Build history of the part. All positions in model axes, mm. Round coordinates to 2 decimals unless told otherwise and drop trailing zeros. Write each loop counter-clockwise with the first axis right and the second up, starting at its lowest first coordinate (ties: lowest second). Pieces come first, ordered by that corner, then holes. Notation, with made-up numbers: (45, -33) -> (62, -33) arc R26 ccw to (62, -17) -> close; hole circle Ø4 at (79, 67.25). An arc over 180 degrees is marked (long way). Answer in a Markdown table with one row per item.
```python
from build123d import *


with BuildPart() as part:
    # Sketch2 → Revolve2 (revolve)
    with BuildSketch(Plane.XY, mode=Mode.PRIVATE) as revolve2_sk:
        with BuildLine():
            ThreePointArc((11.931891232, -1.431891232), (12.525, 0), (11.931891232, 1.431891232))
            Line((11.931891232, 1.431891232), (11.5, 1.863782464))
            Line((11.5, 1.863782464), (11.5, 5.5))
            Line((11.5, 5.5), (16, 5.5))
            Line((16, 5.5), (16, -5.5))
            Line((16, -5.5), (11.5, -5.5))
            Line((11.5, -5.5), (11.5, -1.863782464))
            Line((11.5, -1.863782464), (11.931891232, -1.431891232))
        make_face()
        Polygon((18.4, -3.1), (16, -5.5), (16, 5.5), (18.4, 3.1), align=None)
    revolve(revolve2_sk.sketch.rotate(Axis((0, 0, 0), (0, 1, 0)), 90), axis=Axis((0, 0, 0), (0, 1, 0)))


solid = part.part
```
Q1. Saw through at D-D on y = -4. Write the cut outline in (x, z), plus the area to 3 significant figures.
A:
| item | result |
|---|---|
| outline | circle Ø35 at (0, 0); hole circle Ø23 at (0, 0) |
| area | 547 mm² |
Q2. Saw through at A-A on x = 0. Write the cut outline in (y, z) (3 decimals).
A:
| item | result |
|---|---|
| outline | (-5.5, -16) -> (-3.1, -18.4) -> (3.1, -18.4) -> (5.5, -16) -> (5.5, -11.5) -> (1.864, -11.5) -> (1.432, -11.932) arc R2.025 cw to (-1.432, -11.932) -> (-1.864, -11.5) -> (-5.5, -11.5) -> close; (-5.5, 11.5) -> (-1.864, 11.5) -> (-1.432, 11.932) arc R2.025 cw to (1.432, 11.932) -> (1.864, 11.5) -> (5.5, 11.5) -> (5.5, 16) -> (3.1, 18.4) -> (-3.1, 18.4) -> (-5.5, 16) -> close |
Q3. Drop flat-ended pins along their axis: P1, Ø6, axis at x = -7, z = -3.5, coming from the -Y side; P2, Ø1, axis at x = -8, y = 3.5, coming from the -Z side; P3, Ø4, axis at x = -3.5, y = 1, coming from the -Z side; P4, Ø1.5, axis at x = 12.5, z = 12, coming from the +Y side. Give the stop position or say it passes through.
A:
| item | result |
|---|---|
| P1 | through |
| P2 | z = -16.71 |
| P3 | z = -18.34 |
| P4 | y = 4.92 |
Q4. Saw through at B-B on z = 0. Write the cut outline in (x, y) (3 decimals), plus the area to 3 significant figures.
A:
| item | result |
|---|---|
| outline | (-18.4, -3.1) -> (-16, -5.5) -> (-11.5, -5.5) -> (-11.5, -1.864) -> (-11.932, -1.432) arc R2.025 cw to (-11.932, 1.432) -> (-11.5, 1.864) -> (-11.5, 5.5) -> (-16, 5.5) -> (-18.4, 3.1) -> close; (11.5, -5.5) -> (16, -5.5) -> (18.4, -3.1) -> (18.4, 3.1) -> (16, 5.5) -> (11.5, 5.5) -> (11.5, 1.864) -> (11.932, 1.432) arc R2.025 cw to (11.932, -1.432) -> (11.5, -1.864) -> close |
| area | 135 mm² |
Q5. Wall check: line 1 (X direction, y = -2.65, z = 0); line 2 (Z direction, x = 14, y = -0.5); line 3 (X direction, y = 3.75, z = -2.5). Give the ranges that are in metal, low to high. Write a range as [from, to].
A:
| item | result |
|---|---|
| line 1 | [-18.4, -11.5], [11.5, 18.4] |
| line 2 | [-11.94, 11.94] |
| line 3 | [-17.57, -11.22], [11.22, 17.57] |
Q6. Saw through at C-C on y = 4.75. Write the cut outline in (x, z).
A:
| item | result |
|---|---|
| outline | circle Ø33.5 at (0, 0); hole circle Ø23 at (0, 0) |
Q7. Two-plate mould, pull along Z, no slides. Class faces 1 (the cylindrical face through (-11.4, 3.7, 1.5)), 2 (the flat face through (-11, 5.5, -4)), 3 (the cylindrical face through (11.2, 0, 14.6)): released by +Z, released by -Z, zero draft, split by the parting line, or undercut.
A:
| item | result |
|---|---|
| face 1 | undercut |
| face 2 | zero draft |
| face 3 | split by the parting line |
